```python
from build123d import *

# Parameters (mm, degrees)
F0_W     = 50
F0_H     = 50
F0_R     = 1.5
F1_DEPTH = 2
F0_R_2   = 0.9
F2_DEPTH = 5
F3_DEPTH = 10


with BuildPart() as f1:
    # F0 (on Top) → F1 (new body)
    with BuildSketch(Plane.XY):
        Rectangle(F0_W, F0_H)
        with Locations((5, -16.156757)):
            Circle(F0_R, mode=Mode.SUBTRACT)
        with Locations((-22, 21.620819)):
            Circle(F0_R, mode=Mode.SUBTRACT)
        with Locations((21, 21.843243)):
            Circle(F0_R, mode=Mode.SUBTRACT)
    extrude(amount=F1_DEPTH)

    # F0 (on Top) → F2 (join)
    with BuildSketch(Plane.XY):
        with Locations((-22, 21.620819)):
            Circle(F0_R)
        with Locations((-22, 21.620819)):
            Circle(F0_R_2, mode=Mode.SUBTRACT)
        with Locations((21, 21.843243)):
            Circle(F0_R)
        with Locations((21, 21.843243)):
            Circle(F0_R_2, mode=Mode.SUBTRACT)
        with Locations((5, -16.156757)):
            Circle(F0_R)
        with Locations((5, -16.156757)):
            Circle(F0_R_2, mode=Mode.SUBTRACT)
    extrude(amount=F2_DEPTH)

    # F0 (on Top) → F3 (join)
    with BuildSketch(Plane.XY):
        with Locations((-22, 21.620819)):
            Circle(F0_R_2)
        with Locations((21, 21.843243)):
            Circle(F0_R_2)
        with Locations((5, -16.156757)):
            Circle(F0_R_2)
    extrude(amount=F3_DEPTH)


solid = f1.part
```
Design review of the part built by this model. Coordinates are the model's own, in mm. A direction names the side the tool comes from. Coordinates: 2 decimals unless noted, no trailing zeros. Loops run counter-clockwise (first coordinate to the right, second up) from the corner with the lowest first, then second, coordinate; pieces in that order, holes last. Notation, with made-up numbers: (61, 89.5) - (84, 89.5) arc R35 ccw to (84, 125.5) - close; hole circle Ø1 at (-11, 63.25). An arc over 180 degrees is marked (long way). Use CSV: the item, a comma, the result in double quotes. Start each with the question number.
1) Consider section C-C on y = 13.5. Write out the cut boundary in (x, z), then the cut area to 3 significant figures.
2) Wall thickness on L1, parallel to Z at x = 16.5, y = -17; L2, parallel to Y at x = 6, z = 3.5; L3, parallel to Y at x = 21.5, z = 9.25: over which ranges is each line inside the solid? List them lowest first. Write a range as from..to.
3) Consider section D-D on z = 7. Write out the cut boundary in (x, y), then the cut area to 3 significant figures.
4) Consider section B-B on z = 3. Write out the cut boundary in (x, y).
5) Consider section A-A on x = 5. Write out the cut boundary in (y, z), then the cut area to 3 significant figures.
6) The part is to be moulded in two halves that separate along X. For faces 1 (the cylindrical face through (5.806, -14.892, 3.479)), 2 (the flat face through (22, 21, 5)), 3 (the flat face through (6, -17, 5)), say which applies: +X half, -X half, draft (parallel to the pull), parting line (faces both ways), or undercut.
7) For pin 1 Ø3 at (y, z) = (-4, 4.5) entering from -X; pin 2 Ø6 at (y, z) = (-18.5, 7.5) entering from -X; pin 3 Ø8 at (x, y) = (-12.5, -4) entering from +Z, all flat-tipped, find the tip position at first contact; note any pin that passes through.
8) Tool access review of faces 4 (the cylindrical face through (20.883, 22.736, 7.465)), 5 (the flat face through (-25, 0, 1)): name each direction out of +Z, -Z, +X, -X, +Y, -Y from which nothing blocks a thin tool from reaching the whole face with its end or side.
Geometry says:
1,outline,"(-25, 0) - (25, 0) - (25, 2) - (-25, 2) - close"
1,area,"100 mm^2"
2,L1,"0..2"
2,L2,"-17.27..-15.04"
2,L3,"21.09..22.59"
3,outline,"circle Ø1.8 at (-22, 21.62); circle Ø1.8 at (5, -16.16); circle Ø1.8 at (21, 21.84)"
3,area,"7.63 mm^2"
4,outline,"circle Ø3 at (-22, 21.62); circle Ø3 at (5, -16.16); circle Ø3 at (21, 21.84)"
5,outline,"(-25, 0) - (25, 0) - (25, 2) - (-14.66, 2) - (-14.66, 5) - (-15.26, 5) - (-15.26, 10) - (-17.06, 10) - (-17.06, 5) - (-17.66, 5) - (-17.66, 2) - (-25, 2) - close"
5,area,"118 mm^2"
6,face 1,"parting line"
6,face 2,"undercut"
6,face 3,"draft"
7,pin 1,"through"
7,pin 2,"x = 3.67"
7,pin 3,"z = 2"
8,face 4,"+Z"
8,face 5,"+Z, -Z, -X, +Y, -Y"
